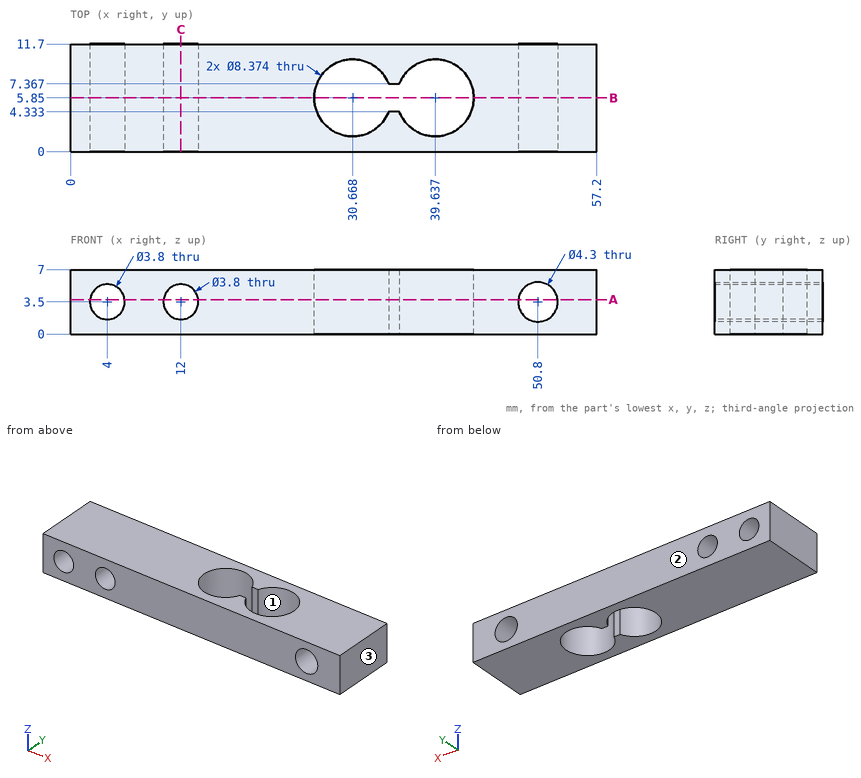
Design review of the part shown in the three views and the two pictorial views. Dimensions are in mm from the part's minimum x, y and z. Give positions to 0.01 mm unless a question says otherwise; leave off trailing zeros. Loops run counter-clockwise (first coordinate to the right, second up) from the corner with the lowest first, then second, coordinate; pieces in that order, holes last. Notation, with made-up numbers: M 10.25,27.5 L 50.25,27.5 A17 cw 50.25,49.5 Z; hole C 56.5,50 d1. An arc over 180 degrees is marked long. Put each result on its own line as item: value. Start each with the question number.
(1) Add section A-A, the plane z = 3.75. Give the number of separate pieces and of enclosed holes in the cut face.
(2) Add section C-C, the plane x = 12. Write out the cut boundary in (y, z).
(3) Add section B-B, the plane y = 5.85. Write out the cut boundary in (x, z), then the cut area to 3 significant figures.
(4) Wall thickness on L1, parallel to X at y = 6, z = 6.25 (1 decimal); L2, parallel to Z at x = 4, y = 7; L3, parallel to X at y = 0.5, z = 3: over which ranges is each line inside the solid? List them lowest first.
(5) For pin 1 (1 mm diameter, centred on x = 50.5, z = 4.5, fed in from -Y), flat-tipped, find the tip position at first contact; note if it passes through.
(6) The part is to be moulded in two halves that separate along Y. For the marked faces 1, 2 and 3, say which applies: +Y half, -Y half, draft (parallel to the pull), parting line (faces both ways), or undercut.
Result:
1. separate pieces: 4
1. enclosed holes: 1
2. outline: M 0,0 L 11.7,0 L 11.7,1.6 L 0,1.6 Z; M 0,5.4 L 11.7,5.4 L 11.7,7 L 0,7 Z
3. outline: M 0,0 L 26.48,0 L 26.48,7 L 0,7 Z; M 43.82,0 L 57.2,0 L 57.2,7 L 43.82,7 Z; hole C 4,3.5 d3.8; hole C 12,3.5 d3.8; hole C 50.8,3.5 d4.3
3. area: 242 mm^2
4. L1: x = 0 to 26.5, 43.8 to 57.2
4. L2: z = 0 to 1.6, 5.4 to 7
4. L3: x = 0 to 2.17, 5.83 to 10.17, 13.83 to 48.71, 52.89 to 57.2
5. pin 1: passes through
6. face 1: undercut
6. face 2: +Y half
6. face 3: draft
